The drawing under review shows one solid part. Ordinate dimensions are in mm from its lowest x, y, z. A direction names the side the tool comes from. Coordinates: 2 decimals unless noted, no trailing zeros. Loops run counter-clockwise (first coordinate to the right, second up) from the corner with the lowest first, then second, coordinate; pieces in that order, holes last. Notation, with made-up numbers: M -2,53.5 L 31,53.5 A22 ccw 31,73.5 Z; hole C -10,13 d9. An arc over 180 degrees is marked long. Use one line per item in the form item = value.
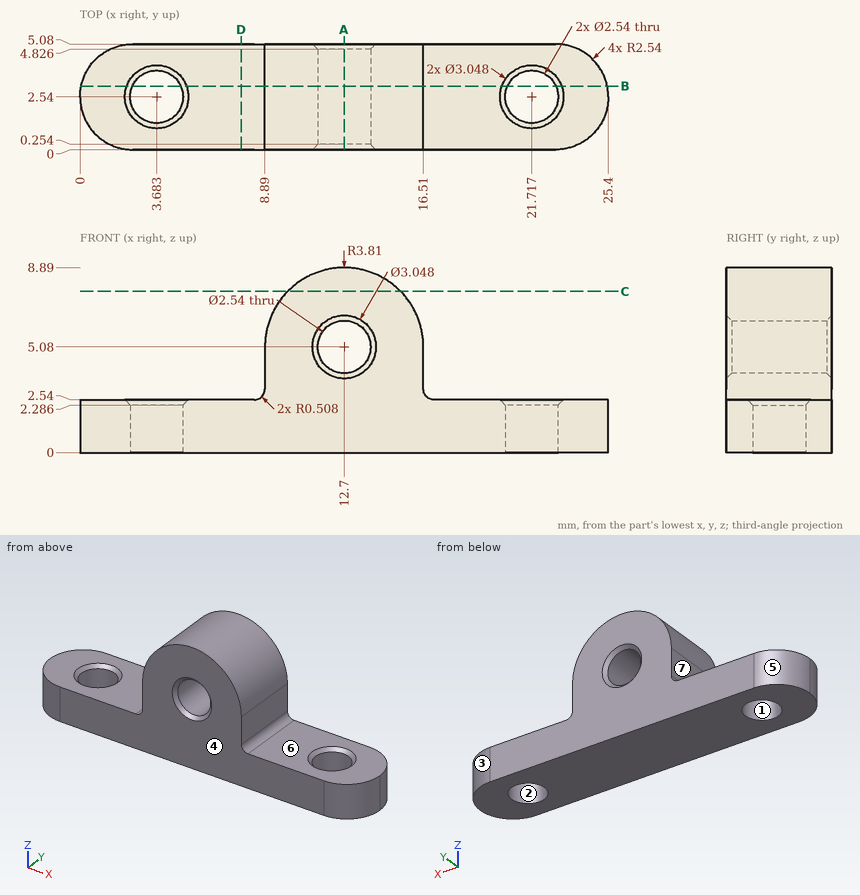
1. For pin 1 Ø1.5 at (x, y) = (19.5, 1.5) entering from +Z; pin 2 Ø0.6 at (y, z) = (3.5, 4.5) entering from +X; pin 3 Ø0.6 at (y, z) = (1.5, 4) entering from -X; pin 4 Ø2 at (x, y) = (3.683, 2.54) entering from +Z, all flat-tipped, find the tip position at first contact; note any pin that passes through.
Computed values:
pin_1 = 2.54
pin_2 = 16.51
pin_3 = 8.89
pin_4 = through
2. Consider section D-D on x = 7.75. Write out the cut boundary in (y, z).
Computed values:
outline = M 0,0 L 5.08,0 L 5.08,2.54 L 0,2.54 Z
3. Draft analysis for pull direction Y (two halves, no side actions). For the marked faces 1, 2, 3 and 4, state which applies: +Y half, -Y half, draft (parallel to the pull), parting line (faces both ways), or undercut.
Computed values:
face_1 = undercut
face_2 = undercut
face_3 = +Y half
face_4 = -Y half
4. Consider section C-C on z = 7.75. Write out the cut boundary in (x, y).
Computed values:
outline = M 9.98,0 L 15.42,0 L 15.42,5.08 L 9.98,5.08 Z
5. Consider section B-B on y = 3.05. State how many separate pieces and enclosed holes the cut face has, plus the area to 3 significant figures.
Computed values:
separate_pieces = 3
enclosed_holes = 1
area = 89.5 mm2
6. Wall thickness on line 1 along X through (y, z) = (3.2, 5.08); line 2 along Z through (x, y) = (18, 3.75); line 3 along X through (y, z) = (3.1, 5.5): over which ranges is each line inside the solid? List them lowest first. Write a range as from..to.
Computed values:
line_1 = 8.89..11.43, 13.97..16.51
line_2 = 0..2.54
line_3 = 8.91..11.5, 13.9..16.49
7. Consider section A-A on x = 12.7. Write out the cut boundary in (y, z).
Computed values:
outline = M 0,0 L 5.08,0 L 5.08,3.56 L 4.83,3.81 L 0.25,3.81 L 0,3.56 Z; M 0,6.6 L 0.25,6.35 L 4.83,6.35 L 5.08,6.6 L 5.08,8.89 L 0,8.89 Z
8. Tool access review of the marked faces 5, 6 and 7: name each direction out of +Z, -Z, +X, -X, +Y, -Y from which nothing blocks a thin tool from reaching the whole face with its end or side.
Computed values:
face_5 = +Z, -Z, -X, +Y
face_6 = +Z, +X, +Y, -Y
face_7 = +Z, -X, +Y, -Y
